Here's the drawing with two shaded views (mm, measured from the low corner). I have some questions. A direction names the side the tool comes from. Coordinates: 2 decimals unless noted, no trailing zeros. Write each loop counter-clockwise with the first axis right and the second up, starting at its lowest first coordinate (ties: lowest second). Pieces come first, ordered by that corner, then holes. Notation, with made-up numbers: (7, 76) -> (22, 76) arc R20 ccw to (22, 84) -> close; hole circle Ø8 at (83, 28.5). An arc over 180 degrees is marked (long way). Put each result on its own line as item: value. Start each with the question number.
Item 1: I want a section at A-A, the plane y = 54. List the corners of the cut face in (x, z) for me.
Item 2: For pin 1 (1 mm diameter, centred on y = 21.5, z = 27, fed in from +X); pin 2 (14.5 mm diameter, centred on y = 59.5, z = 11, fed in from +X); pin 3 (6 mm diameter, centred on y = 3.5, z = 29, fed in from -X); pin 4 (1 mm diameter, centred on x = 13, y = 21.5, fed in from -Z), each with a flat end and sliding along its axis, tell me the tip position at first contact or that it passes through.
Item 3: I need wall thicknesses on line 1 (X direction, y = 59, z = 27); line 2 (Z direction, x = 12, y = 34); line 3 (Y direction, x = 60.5, z = 5). Which ranges of each line are inside material? Lowest first, please. Write a range as [from, to].
Item 4: I want a section at B-B, the plane x = 40. List the corners of the cut face in (y, z) for me.
Item 5: On a 3-axis mill with a long thin cutter (end or side, diameter ignored), from which of +Z, -Z, +X, -X, +Y, -Y can I reach the whole of each face in a straight line? I mean the marked faces 4, 5, 6, 7 and 8. Say none if no direction works.
Item 6: If we mould it in two halves opening along Y, with no side actions, what happens to the marked faces 1, 2 and 3? For each: released by +Y, released by -Y, zero draft, split by the parting line, or undercut.
Item 7: I want a section at C-C, the plane z = 4. List the corners of the cut face in (x, y) for me.
Item 8: I want a section at D-D, the plane y = 16.5. List the corners of the cut face in (x, z) for me, then the cut area to 3 significant figures.
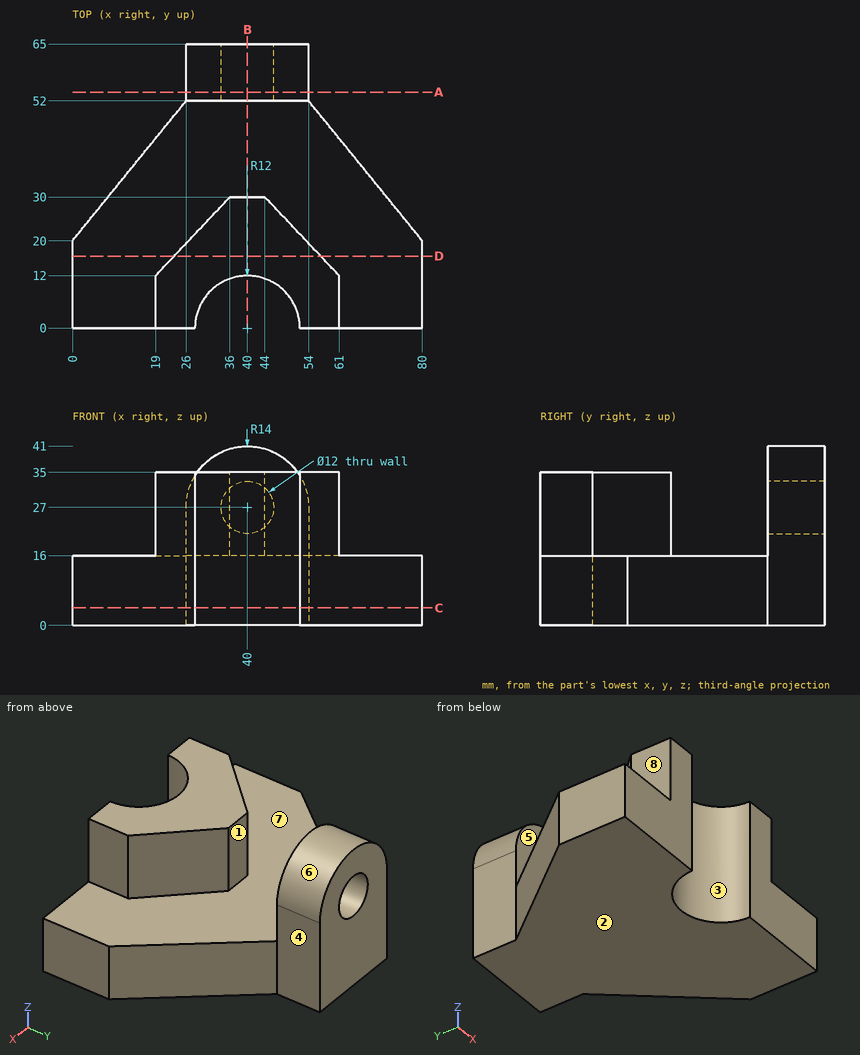
Calculated:
1. outline: (26, 0) -> (54, 0) -> (54, 27) arc R14 ccw to (26, 27) -> close; hole circle Ø12 at (40, 27)
2. pin 1: stops at x = 52.5
2. pin 2: stops at x = 54
2. pin 3: stops at x = 19
2. pin 4: stops at z = 0
3. line 1: x = [26, 34], [46, 54]
3. line 2: z = [0, 16]
3. line 3: y = [0, 44]
4. outline: (12, 0) -> (65, 0) -> (65, 21) -> (52, 21) -> (52, 16) -> (30, 16) -> (30, 35) -> (12, 35) -> close; (52, 33) -> (65, 33) -> (65, 41) -> (52, 41) -> close
5. face 4: +Z, -Z, +X, +Y
5. face 5: +Z, +X, -X
5. face 6: +Z, +Y
5. face 7: +Z
5. face 8: +Z, -X, +Y, -Y
6. face 1: undercut
6. face 2: zero draft
6. face 3: released by -Y
7. outline: (0, 0) -> (28, 0) arc R12 cw to (52, 0) -> (80, 0) -> (80, 20) -> (54, 52) -> (54, 65) -> (26, 65) -> (26, 52) -> (0, 20) -> close
8. outline: (0, 0) -> (80, 0) -> (80, 16) -> (56.75, 16) -> (56.75, 35) -> (23.25, 35) -> (23.25, 16) -> (0, 16) -> close
8. area: 1,920 mm2
